Could you check a few things on this model? Use its own coordinates, in mm. A direction names the side the tool comes from. Round coordinates to 2 decimals unless told otherwise and drop trailing zeros. Loops run counter-clockwise (first coordinate to the right, second up) from the corner with the lowest first, then second, coordinate; pieces in that order, holes last. Notation, with made-up numbers: (82, -14.75) -> (114, -14.75) arc R23 cw to (114, 13.25) -> close; hole circle Ø7 at (7, -6.75). An arc over 180 degrees is marked (long way). One line per item, written item: value.
from build123d import *

# Parameters (mm, degrees)
F0_W     = 12.7
F0_H     = 6.35
F0_W_2   = 6.35
F0_H_2   = 38.1
F0_H_3   = 2.4236633693
F2_SIZE2 = 8.89
F2_SIZE  = 17.78
F3_SIZE2 = 0.508
F3_SIZE  = 1.27


with BuildPart() as f1:
    # F0 (on Front) → F1 (revolve)
    with BuildSketch(Plane.XZ):
        with Locations((-19.05, -28.2841619736)):
            Rectangle(F0_W, F0_H)
        with Locations((-9.525, -6.0591619736)):
            Rectangle(F0_W_2, F0_H_2)
        with Locations((-9.525, -28.2841619736)):
            Rectangle(F0_W_2, F0_H)
        with Locations((-9.525, 14.2026697111)):
            Rectangle(F0_W_2, F0_H_3)
        with Locations((-19.05, 14.2026697111)):
            Rectangle(F0_W, F0_H_3)
        Polygon((-25.4, 15.4145013957), (-12.7, 15.4145013957), (-6.35, 15.4145013957), (-6.35, 19.3408380264), (-25.4, 19.3408380264), align=None)
    revolve(axis=Axis((0, 0, 6.5382700413), (0, 0, -1)))

    # F2
    f2_edges = [f1.edges().sort_by_distance(p)[0] for p in [
        (12.7, 0, 12.990838),
        (12.7, 0, -25.109162),
    ]]
    f2_side = f1.faces().sort_by_distance((12.7, 0, -6.059162))[0]
    chamfer(f2_edges, length=F2_SIZE, length2=F2_SIZE2, reference=f2_side)

    # F3
    f3_edges = [f1.edges().sort_by_distance(p)[0] for p in [
        (25.4, 0, -31.459162),
    ]]
    f3_side = f1.faces().sort_by_distance((24.68158, 0, -31.459162))[0]
    chamfer(f3_edges, length=F3_SIZE, length2=F3_SIZE2, reference=f3_side)


solid = f1.part
(1) If I drill on L1, parallel to Z at x = -10, y = 19.5; L2, parallel to Y at x = 0, z = -7; L3, parallel to Z at x = -19.5, y = 5.5, over which ranges is the centre line in solid material (lowest first)?
Recorded:
L1: -31.46 to -25.11, 12.99 to 19.34
L2: -12.7 to -6.35, 6.35 to 12.7
L3: -31.46 to -22.45, 10.33 to 19.34
(2) If we section it at C-C, the plane z = 4: Please give me the cut outline in (x, y), then the cut area to 3 significant figures.
Recorded:
outline: circle Ø34.19 at (0, 0); hole circle Ø12.7 at (0, 0)
area: 791 mm²
(3) Thinking about a two-plate mould opening in Z: for faces 1 (the face through (0.8, 6.3, -5.7)), 2 (the face through (11.303, -8.667, -10.417)), 3 (the face through (5, -5, 19.341)), which applies, released by +Z, released by -Z, zero draft, split by the parting line, or undercut?
Recorded:
face 1: zero draft
face 2: undercut
face 3: released by +Z
(4) For faces 4 (the face through (5.506, -24.796, 16.121)), 5 (the face through (11, -19, -25.109)), which set-ups out of +Z, -Z, +X, -X, +Y, -Y let a thin tool reach every point of the face, with its end or its side?
Recorded:
face 4: +Z, -Z
face 5: none
(5) I'm going to push flat-ended pins straight in: pin 1 Ø8 at (x, z) = (-16, -4.5) entering from +Y; pin 2 Ø5 at (y, z) = (17, -17.5) entering from -X; pin 3 Ø3 at (y, z) = (6, 12) entering from +X. Where does each tip first touch, or does it pass through?
Recorded:
pin 1: y = 5.88
pin 2: x = -10.9
pin 3: x = 24.93
(6) If we section it at A-A, the plane x = 0: Please give me the cut outline in (y, z).
Recorded:
outline: (-25.4, -30.95) -> (-24.13, -31.46) -> (-6.35, -31.46) -> (-6.35, 19.34) -> (-25.4, 19.34) -> (-25.4, 12.99) -> (-21.59, 12.99) -> (-12.7, -4.79) -> (-12.7, -7.33) -> (-21.59, -25.11) -> (-25.4, -25.11) -> close; (6.35, -31.46) -> (24.13, -31.46) -> (25.4, -30.95) -> (25.4, -25.11) -> (21.59, -25.11) -> (12.7, -7.33) -> (12.7, -4.79) -> (21.59, 12.99) -> (25.4, 12.99) -> (25.4, 19.34) -> (6.35, 19.34) -> close
(7) If we section it at D-D, the plane z = -2.5: Please give me the cut outline in (x, y), then the cut area to 3 significant figures.
Recorded:
outline: circle Ø27.69 at (0, 0); hole circle Ø12.7 at (0, 0)
area: 475 mm²
